Model file for the job. Use its own axes, mm. A direction names the side the tool comes from. Coordinates: 2 decimals unless noted, no trailing zeros. Write each loop counter-clockwise with the first axis right and the second up, starting at its lowest first coordinate (ties: lowest second). Pieces come first, ordered by that corner, then holes.
Q1. Which spindle directions (+Z, -Z, +X, -X, +Y, -Y) get a long thin tool onto all of the face, cutting with end or side? Do faces 1 (the flat face through (-1.25, -1, 26)), 2 (the flat face through (1.25, -1, 26)), 3 (the flat face through (-1, 1, 0)). Say none if no direction does.
Q2. Pin check, flat tips, straight feed: P1, Ø10, axis at x = 10.5, z = 35.5, coming from the +Y side; P2, Ø1.2, axis at x = 0, y = 35.5, coming from the -Z side; P3, Ø2, axis at x = 0.5, z = 23, coming from the +Y side; P4, Ø1.2, axis at x = -0.5, z = 30, coming from the -Y side. Stop position of each tip, or through.
Q3. Band-saw the part on C-C, the plane x = -40. Write the cut outline in (y, z), plus the area to 3 significant figures.
Q4. Band-saw the part on B-B, the plane y = -56.5. Write the cut outline in (x, z), plus the area to 3 significant figures.
Q5. Band-saw the part on D-D, the plane x = 6. Write the cut outline in (y, z).
Q6. Band-saw the part on A-A, the plane y = 0. Write the cut outline in (x, z).
Q7. Drill centre lines: probe 1 along Z at (x, y) = (-0.7, -20.6); probe 2 along Z at (x, y) = (-54, -30.5); probe 3 along X at (y, z) = (-4, 17.5). Where is each one in solid material? Low to high.
from build123d import *

# Parameters (mm, degrees)
F0_R     = 100
F0_W     = 7
F0_H     = 60
F0_W_2   = 2.5
F0_H_2   = 180
F1_DEPTH = 2
F2_DEPTH = 50
F3_R     = 1.6
F3_W     = 13
F3_H     = 34
F4_DEPTH = 4
F5_R     = 4


with BuildPart() as f1:
    # F0 (on Top) → F1 (new body)
    with BuildSketch(Plane.XY):
        Circle(F0_R)
        with Locations((-26.5, 0)):
            Rectangle(F0_W, F0_H, mode=Mode.SUBTRACT)
        Rectangle(F0_W_2, F0_H_2, mode=Mode.SUBTRACT)
        with Locations((26.5, 0)):
            Rectangle(F0_W, F0_H, mode=Mode.SUBTRACT)
    extrude(amount=F1_DEPTH)

    # F0 (on Top) → F2 (join)
    with BuildSketch(Plane.XY):
        Rectangle(F0_W_2, F0_H_2)
    extrude(amount=F2_DEPTH)

    # F3 (on face) → F4 (cut)
    with BuildSketch(Plane.YZ.offset(1.25)):
        with Locations((-20.6, 19.55)):
            Circle(F3_R)
        with Locations((20.6, 19.55)):
            Circle(F3_R)
        with Locations((-76.5, 26)):
            Rectangle(F3_W, F3_H)
        with Locations((-56.5, 26)):
            Rectangle(F3_W, F3_H)
        with Locations((-36.5, 26)):
            Rectangle(F3_W, F3_H)
        with Locations((76.5, 26)):
            Rectangle(F3_W, F3_H)
        with Locations((56.5, 26)):
            Rectangle(F3_W, F3_H)
        with Locations((36.5, 26)):
            Rectangle(F3_W, F3_H)
    extrude(amount=-F4_DEPTH, mode=Mode.SUBTRACT)

    # F5
    f5_edges = [f1.edges().sort_by_distance(p)[0] for p in [
        (0, -90, 50),
        (0, 90, 50),
        (0, 50, 9),
        (0, 63, 9),
        (0, 83, 9),
        (0, 70, 9),
        (0, 30, 9),
        (0, -43, 9),
        (0, 83, 43),
        (0, 63, 43),
        (0, 43, 43),
        (0, -30, 43),
        (0, -50, 43),
        (0, -70, 43),
        (0, -70, 9),
        (0, -50, 9),
        (0, -30, 9),
        (0, -63, 9),
        (0, -83, 9),
        (0, 70, 43),
        (0, 50, 43),
        (0, 30, 43),
        (0, -63, 43),
        (0, -43, 43),
        (0, -83, 43),
        (0, 43, 9),
    ]]
    fillet(f5_edges, radius=F5_R)


solid = f1.part
Answer sheet:
1. face 1: +Z, -X, +Y, -Y
1. face 2: +Z, +X, +Y, -Y
1. face 3: -Z, +X, -X, +Y, -Y
2. P1: passes through
2. P2: stops at z = 0
2. P3: stops at y = 90
2. P4: stops at y = -90
3. outline: (-91.65, 0) - (91.65, 0) - (91.65, 2) - (-91.65, 2) - close
3. area: 367 mm2
4. outline: (-82.51, 0) - (82.51, 0) - (82.51, 2) - (1.25, 2) - (1.25, 9) - (-1.25, 9) - (-1.25, 2) - (-82.51, 2) - close; (-1.25, 43) - (1.25, 43) - (1.25, 50) - (-1.25, 50) - close
4. area: 365 mm2
5. outline: (-99.82, 0) - (99.82, 0) - (99.82, 2) - (-99.82, 2) - close
6. outline: (-100, 0) - (-30, 0) - (-30, 2) - (-100, 2) - close; (-23, 0) - (23, 0) - (23, 2) - (1.25, 2) - (1.25, 50) - (-1.25, 50) - (-1.25, 2) - (-23, 2) - close; (30, 0) - (100, 0) - (100, 2) - (30, 2) - close
7. probe 1: z = 0 to 17.95, 21.15 to 50
7. probe 2: z = 0 to 2
7. probe 3: x = -1.25 to 1.25
